Solid Edge part; units mm, degrees
sketch "Sketch1" plane through (0, 0, 0) normal (0, 0, 1) x (1, 0, 0)
  line L0 (-57.5, -17) -> (57.5, -17)
  line L1 (57.5, -17) -> (57.5, 17)
  line L2 (57.5, 17) -> (-57.5, 17)
  line L3 (-57.5, 17) -> (-57.5, -17)
extrude "Protrusion1" add sketch "Sketch1" against normal blind 10
sketch "Sketch2" plane through (0, 0, 0) normal (0, 0, 1) x (1, 0, 0)
  line L0 (-57.5, -17) -> (42.5, -17)
  line L1 (42.5, -17) -> (42.5, -7)
  line L2 (42.5, -7) -> (-57.5, -7)
  line L3 (-57.5, -7) -> (-57.5, -17)
extrude "ExtrudedCutout_1" cut sketch "Sketch2" against normal blind 10
sketch "Sketch3" plane through (0, 0, 0) normal (0, 0, 1) x (1, 0, 0)
  line L0 (57.5, 2.2) -> (-57.5, 17)
  line L1 (-57.5, 17) -> (57.5, 17)
  line L2 (57.5, 17) -> (57.5, 2.2)
extrude "ExtrudedCutout_2" cut sketch "Sketch3" against normal blind 10
fillet "Round_1" radius 5 1 edges at (57.5, 2.2, -5)
sketch "Sketch4" plane through (0, 0, 0) normal (0, 0, 1) x (0, 1, 0)
  circle A0 centre (24.0455, -35.6848) radius 22.4024
extrude "ExtrudedCutout_3" cut sketch "Sketch4" against normal blind 10
fillet "Round_2" radius 10 1 edges at (45.2312, 3.7789, -5)
fillet "Round_3" radius 10 1 edges at (21.318, 6.8565, -5)
sketch "Sketch5" plane through (0, 0, 0) normal (0, 0, 1) x (1, 0, 0)
  line L0 (-57.5, -7) -> (-41.5, -7)
  line L1 (-41.5, -7) -> (-41.5, 14.9409)
  line L2 (-41.5, 14.9409) -> (-57.5, 17)
  line L3 (-57.5, 17) -> (-57.5, -7)
extrude "ExtrudedCutout_4" cut sketch "Sketch5" against normal blind 5
fillet "Round_4" radius 10 1 edges at (-41.5, -7, -2.5)
sketch "Sketch6" plane through (-44.5, 5, -5) normal (0, 0, 1) x (1, 0, 0)
  circle A0 centre (-5, 3) radius 2.75
extrude "ExtrudedCutout_6" cut sketch "Sketch6" against normal blind 5.5
fillet "Round_5" radius 10 1 edges at (-57.5, -7, -7.5)
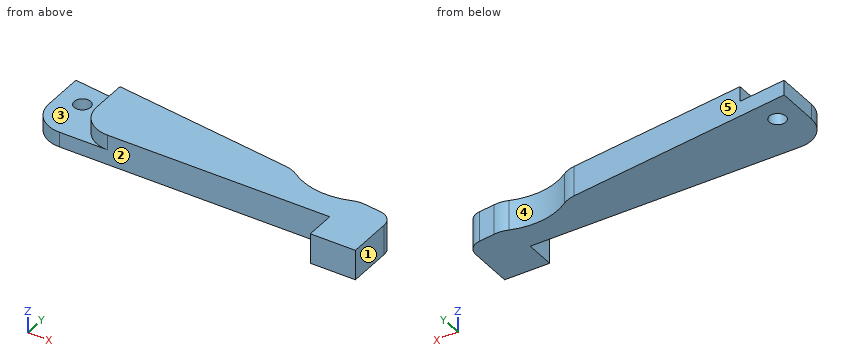
Read the model definition and answer for the solid it produces. Units are mm, in the model's axes. Face numbers are marked on the shaded views. A direction names the side the tool comes from. Give positions to 0.01 mm unless a question says otherwise; leave off trailing zeros. Loops run counter-clockwise (first coordinate to the right, second up) from the corner with the lowest first, then second, coordinate; pieces in that order, holes last. Notation, with made-up numbers: (-22, -39.75) -> (21, -39.75) arc R18 cw to (21, -27.75) -> close; hole circle Ø3 at (70, -19). An arc over 180 degrees is marked (long way). Use a Markdown table: item, result.
Q1. Section D-D, the plane x = -33 is taken. Determine the outline of the cut face in (y, z), then the cut area to 3 significant figures.
Solved:
| item | result |
|---|---|
| outline | (-7, -10) -> (13.85, -10) -> (13.85, 0) -> (-6.89, 0) -> (-6.89, -5) -> (-7, -5) -> close |
| area | 208 mm^2 |
Q2. Section A-A, the plane x = -49.5 is taken. Determine the outline of the cut face in (y, z).
Solved:
| item | result |
|---|---|
| outline | (-6.8, -10) -> (5.25, -10) -> (5.25, -5) -> (-6.8, -5) -> close; (10.75, -10) -> (15.97, -10) -> (15.97, -5) -> (10.75, -5) -> close |
Q3. Determine the mould class of the marked faces 3, 4 and 5 for opening direction X: pulls with the +X half, pulls with the -X half, needs draft (parallel to the pull), parting line crosses it, or undercut.
Solved:
| item | result |
|---|---|
| face 3 | needs draft |
| face 4 | undercut |
| face 5 | pulls with the +X half |
Q4. Each of these flat-tipped pins is pushed along its axis until it touches: pin 1 (1 mm diameter, centred on y = -12.5, z = -7, fed in from -X); pin 2 (6.5 mm diameter, centred on x = -49.5, y = 8, fed in from +Z); pin 3 (2 mm diameter, centred on x = -30, y = 3.5, fed in from +Z); pin 4 (5 mm diameter, centred on x = 11.5, z = -6.5, fed in from -Y). Where does it stop, or does it pass through?
Solved:
| item | result |
|---|---|
| pin 1 | stops at x = 42.5 |
| pin 2 | stops at z = -5 |
| pin 3 | stops at z = 0 |
| pin 4 | stops at y = -7 |
Q5. A tool of negligible diameter and unlimited length cuts with its end or side. For the marked faces 1 and 2, from which of +Z, -Z, +X, -X, +Y, -Y can it reach the whole face along a straight path? Write none if from no direction.
Solved:
| item | result |
|---|---|
| face 1 | +Z, -Z, +X, +Y, -Y |
| face 2 | +Z, -Z, -X, -Y |
Q6. Section C-C, the plane z = -3 is taken. Determine the outline of the cut face in (x, y).
Solved:
| item | result |
|---|---|
| outline | (-41.5, 3) arc R10 ccw to (-31.5, -7) -> (42.5, -7) -> (42.5, -17) -> (57.5, -17) -> (57.5, -2.2) arc R5 ccw to (53.14, 2.76) -> (47.84, 3.44) arc R10 ccw to (43.21, 2.94) arc R22.4 cw to (23.06, 5.54) arc R10 ccw to (18.71, 7.19) -> (-41.5, 14.94) -> close |
Q7. Section B-B, the plane z = -8 is taken. Determine the outline of the cut face in (x, y), then the cut area to 3 significant figures.
Solved:
| item | result |
|---|---|
| outline | (-57.5, 3) arc R10 ccw to (-47.5, -7) -> (42.5, -7) -> (42.5, -17) -> (57.5, -17) -> (57.5, -2.2) arc R5 ccw to (53.14, 2.76) -> (47.84, 3.44) arc R10 ccw to (43.21, 2.94) arc R22.4 cw to (23.06, 5.54) arc R10 ccw to (18.71, 7.19) -> (-57.5, 17) -> close; hole circle Ø5.5 at (-49.5, 8) |
| area | 1,950 mm^2 |
Q8. Find the intervals of material crossed by line 1 along Y through (x, z) = (-49.5, -7.2); line 2 along X through (y, z) = (-14, -0.5); line 3 along Z through (x, y) = (-42, 13.5), in increasing order.
Solved:
| item | result |
|---|---|
| line 1 | y = -6.8 to 5.25, 10.75 to 15.97 |
| line 2 | x = 42.5 to 57.5 |
| line 3 | z = -10 to -5 |
